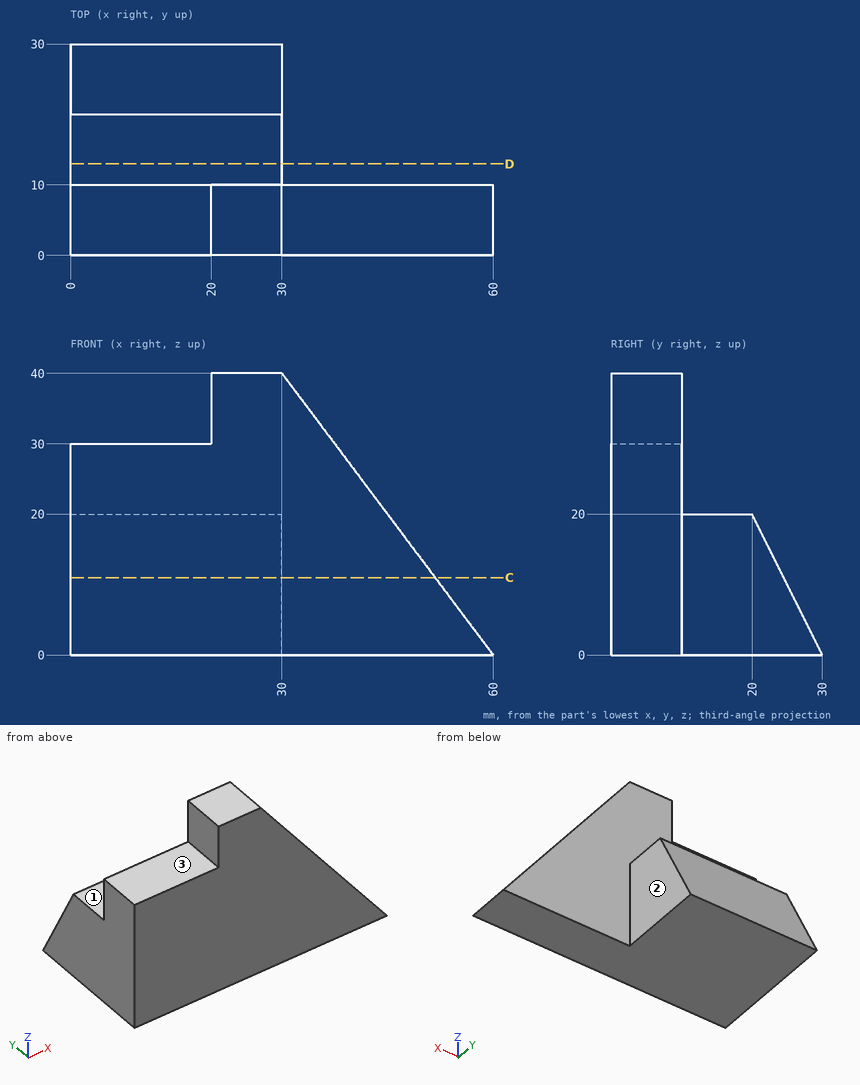
Design review of the part shown in the three views and the two pictorial views. Dimensions are in mm from the part's minimum x, y and z. A direction names the side the tool comes from. Give positions to 0.01 mm unless a question says otherwise; leave off trailing zeros. Loops run counter-clockwise (first coordinate to the right, second up) from the corner with the lowest first, then second, coordinate; pieces in that order, holes last. Notation, with made-up numbers: M 14.25,68 L 45.25,68 A35 ccw 45.25,106 Z; hole C -2.75,-8 d8. An arc over 180 degrees is marked long. Answer as a JSON object with one key per item and string values. Group by question number.
Q1. Insertion check: P1, Ø3, axis at y = 5.5, z = 35, coming from the -X side; P2, Ø12, axis at x = 27.5, z = 14.5, coming from the +Y side; P3, Ø6, axis at x = 6, y = 27, coming from the +Z side. Each pin has a flat end and moves straight along its axis. Give the tip position at first contact, or say it passes through.
Q2. Tool access review of the marked faces 1, 2 and 3: name each direction out of +Z, -Z, +X, -X, +Y, -Y from which nothing blocks a thin tool from reaching the whole face with its end or side.
Q3. Add section C-C on z = 11. Give the boundary of the cut face in (x, y).
Q4. For probe 1 along Y at (x, z) = (52, 10); probe 2 along X at (y, z) = (24.5, 8); probe 3 along Z at (x, y) = (22, 12.5), list the stretches that pass through material, from the lowest coordinate up. Write a range as [from, to].
Q5. Add section D-D on y = 13. Give the boundary of the cut face in (x, z).
Checked values:
{
 "1": {"P1": "x = 20", "P2": "y = 25.75", "P3": "z = 12"},
 "2": {"face 1": "+Z, +X, -X, +Y", "face 2": "+Z, -Z, +X, +Y", "face 3": "+Z, -X, +Y, -Y"},
 "3": {"outline": "M 0,0 L 51.75,0 L 51.75,10 L 30,10 L 30,24.5 L 0,24.5 Z"},
 "4": {"probe 1": "[0, 10]", "probe 2": "[0, 30]", "probe 3": "[0, 20]"},
 "5": {"outline": "M 0,0 L 30,0 L 30,20 L 0,20 Z"}
}
